Could you check a few things on this model? Use its own coordinates, in mm. A direction names the side the tool comes from. Round coordinates to 2 decimals unless told otherwise and drop trailing zeros. Write each loop counter-clockwise with the first axis right and the second up, starting at its lowest first coordinate (ties: lowest second). Pieces come first, ordered by that corner, then holes. Notation, with made-up numbers: (-10, -29.5) - (39, -29.5) arc R31 ccw to (39, -5.5) - close; hole circle Ø3 at (31, 87.25). An arc over 180 degrees is marked (long way). Write each question's results on one line, items separated by ' | '. Start each with the question number.
(1) Imagine slicing it at B-B on z = -2. Write out the boundary of the cut face in (x, y).
(2) For P1, Ø4, axis at y = 8.5, z = -6, coming from the +X side; P2, Ø4.5, axis at x = 6, z = -6.5, coming from the -Y side; P3, Ø1.5, axis at y = 13.5, z = -2, coming from the -X side; P4, Ø6, axis at y = 5, z = 7.5, coming from the +X side, each with a flat end and sliding along its axis, tell me the tip position at first contact or that it passes through.
(3) Imagine slicing it at D-D on z = -10.25. Write out the boundary of the cut face in (x, y).
(4) Imagine slicing it at C-C on x = 18.5. Write out the boundary of the cut face in (y, z), then the cut area to 3 significant figures.
(5) Thinking about a two-plate mould opening in X: for faces 1 (the cylindrical face through (19.5, 13.1, 11.5)), 2 (the flat face through (-15, 14, 10)), 3 (the flat face through (9, 7, 0)), which applies, +X half, -X half, draft (parallel to the pull), parting line (faces both ways), or undercut?
(6) Imagine slicing it at A-A on y = 8. Write out the boundary of the cut face in (x, z).
(7) Please list where these lines run through material, in increasing order: line 1 (X direction, y = 2.15, z = -2); line 2 (Z direction, x = -18.5, y = 0.95); line 3 (X direction, y = 2.75, z = 2). Write a range as [from, to].
(8) On a 3-axis mill with a long thin cutter (end or side, diameter ignored), from which of +Z, -Z, +X, -X, +Y, -Y can I reach the whole of each face in a straight line? I mean faces 4 (the flat face through (-14, 10, 12)), 5 (the flat face through (6, 15, -11)), 6 (the flat face through (-16, 3, -3)), 7 (the flat face through (17, 3, -3)), 8 (the flat face through (-3, 13, 0)). Say none if no direction works.
```python
from build123d import *

# Parameters (mm, degrees)
EXTRU_MINCE1_DEPTH      = 13
EXTRUSION1_DEPTH        = 3
ESQUISSE3_R             = 1.5
ENL_V_MAT_EXTRU_1_DEPTH = 3
ENL_V_MAT_EXTRU_2_REACH = 18
ESQUISSE4_W             = 4
ESQUISSE4_H             = 8
ESQUISSE4_H_2           = 2
ESQUISSE6_W             = 7
ESQUISSE6_H             = 5
ENL_V_MAT_EXTRU_4_DEPTH = 42
ESQUISSE7_R             = 1.5
ENL_V_MAT_EXTRU_5_DEPTH = 3
ESQUISSE8_W             = 4
ESQUISSE8_H             = 16
ENL_V_MAT_EXTRU_6_DEPTH = 1


with BuildPart() as part:
    # Esquisse1 → Extru.-Mince1 (new body, symmetric)
    with BuildSketch(Plane.XY):
        Polygon((-21, 0), (-9, 0), (-9, 13), (9, 13), (9, 0), (21, 0), (21, 3), (12, 3), (12, 16), (-12, 16), (-12, 3), (-21, 3), align=None)
    extrude(amount=EXTRU_MINCE1_DEPTH, both=True)

    # Esquisse2 → Extrusion1 (add)
    with BuildSketch(Plane.XY.offset(13)):
        with BuildLine():
            Line((-12, 16), (-16.5, 16))
            ThreePointArc((-16.5, 16), (-19.5, 13), (-16.5, 10))
            Line((-16.5, 10), (-12, 10))
            Line((-12, 10), (-12, 16))
        make_face()
    extrusion1 = extrude(amount=-EXTRUSION1_DEPTH)

    # Esquisse3 → Enlèv. mat.-Extru.1 (cut)
    with BuildSketch(Plane.XY.offset(13)):
        with Locations((-16.5, 13)):
            Circle(ESQUISSE3_R)
    enl_v_mat_extru_1 = extrude(amount=-ENL_V_MAT_EXTRU_1_DEPTH, mode=Mode.SUBTRACT)

    # Symétrie1: Extrusion1, Enlèv. mat.-Extru.1 across plane
    add(extrusion1.mirror(Plane(origin=(0, 0, 0), x_dir=(0, 0, 1), z_dir=(1, 0, 0))))
    add(enl_v_mat_extru_1.mirror(Plane(origin=(0, 0, 0), x_dir=(0, 0, 1), z_dir=(1, 0, 0))), mode=Mode.SUBTRACT)

    # Esquisse4 → Enlèv. mat.-Extru.2 (cut, up to next)
    with BuildSketch(Plane(origin=(0, 16, 0), x_dir=(1, 0, 0), z_dir=(0, 1, 0)), mode=Mode.PRIVATE) as enl_v_mat_extru_2_sk1:
        with Locations((6, -9)):
            Rectangle(ESQUISSE4_W, ESQUISSE4_H)
    enl_v_mat_extru_2_tool1 = extrude(enl_v_mat_extru_2_sk1.sketch, amount=-ENL_V_MAT_EXTRU_2_REACH, mode=Mode.PRIVATE) & part.part
    add(enl_v_mat_extru_2_tool1.solids().sort_by_distance((6, 16, 9))[0], mode=Mode.SUBTRACT)
    # Esquisse4 → Enlèv. mat.-Extru.2 (cut, up to next)
    with BuildSketch(Plane(origin=(0, 16, 0), x_dir=(1, 0, 0), z_dir=(0, 1, 0)), mode=Mode.PRIVATE) as enl_v_mat_extru_2_sk2:
        with Locations((6, 12)):
            Rectangle(ESQUISSE4_W, ESQUISSE4_H_2)
    enl_v_mat_extru_2_tool2 = extrude(enl_v_mat_extru_2_sk2.sketch, amount=-ENL_V_MAT_EXTRU_2_REACH, mode=Mode.PRIVATE) & part.part
    add(enl_v_mat_extru_2_tool2.solids().sort_by_distance((6, 16, -12))[0], mode=Mode.SUBTRACT)

    # Esquisse6 → Enlèv. mat.-Extru.4 (cut)
    with BuildSketch(Plane(origin=(21, 0, 0), x_dir=(0, 0, -1), z_dir=(1, 0, 0))):
        with Locations((-9.5, 2.5)):
            Rectangle(ESQUISSE6_W, ESQUISSE6_H)
    extrude(amount=-ENL_V_MAT_EXTRU_4_DEPTH, mode=Mode.SUBTRACT)

    # Esquisse7 → Enlèv. mat.-Extru.5 (cut)
    with BuildSketch(Plane(origin=(0, 3, 0), x_dir=(1, 0, 0), z_dir=(0, 1, 0))):
        with Locations((18.5, 2)):
            Circle(ESQUISSE7_R)
    enl_v_mat_extru_5 = extrude(amount=-ENL_V_MAT_EXTRU_5_DEPTH, mode=Mode.SUBTRACT)

    # Symétrie2: Enlèv. mat.-Extru.5 across plane
    add(enl_v_mat_extru_5.mirror(Plane(origin=(0, 0, 0), x_dir=(0, 0, 1), z_dir=(1, 0, 0))), mode=Mode.SUBTRACT)

    # Esquisse8 → Enlèv. mat.-Extru.6 (cut)
    with BuildSketch(Plane.XZ.offset(-13)):
        with Locations((6, -3)):
            Rectangle(ESQUISSE8_W, ESQUISSE8_H)
    extrude(amount=-ENL_V_MAT_EXTRU_6_DEPTH, mode=Mode.SUBTRACT)


solid = part.part
```
Response:
1) outline: (-21, 0) - (-20, 0) - (-20, 3) - (-21, 3) - close; (-17, 0) - (-9, 0) - (-9, 13) - (4, 13) - (4, 14) - (8, 14) - (8, 13) - (9, 13) - (9, 0) - (17, 0) - (17, 3) - (12, 3) - (12, 16) - (-12, 16) - (-12, 3) - (-17, 3) - close; (20, 0) - (21, 0) - (21, 3) - (20, 3) - close
2) P1: x = 12 | P2: y = 13 | P3: x = -12 | P4: x = 21
3) outline: (-21, 0) - (-9, 0) - (-9, 13) - (4, 13) - (4, 14) - (8, 14) - (8, 13) - (9, 13) - (9, 0) - (21, 0) - (21, 3) - (12, 3) - (12, 16) - (-12, 16) - (-12, 3) - (-21, 3) - close
4) outline: (0, -13) - (3, -13) - (3, -3.5) - (0, -3.5) - close; (0, -0.5) - (3, -0.5) - (3, 6) - (0, 6) - close; (10.76, 10) - (15.24, 10) - (15.24, 13) - (10.76, 13) - close | area: 61.4 mm²
5) face 1: +X half | face 2: draft | face 3: undercut
6) outline: (-12, -13) - (-9, -13) - (-9, 13) - (-12, 13) - close; (9, -13) - (12, -13) - (12, 13) - (9, 13) - close
7) line 1: [-21, -20], [-17, -9], [9, 17], [20, 21] | line 2: [-13, -3.5], [-0.5, 6] | line 3: [-21, -9], [9, 21]
8) face 4: +Z, -Z, -X, -Y | face 5: -Z, +Y, -Y | face 6: +Z, -Z, -X, +Y | face 7: +Z, -Z, +X, +Y | face 8: +Z, -Z, -Y
